Verification items for the finished model (mm, model axes). A direction names the side the tool comes from. Coordinates: 2 decimals unless noted, no trailing zeros. Loops run counter-clockwise (first coordinate to the right, second up) from the corner with the lowest first, then second, coordinate; pieces in that order, holes last. Notation, with made-up numbers: (51.5, 15) - (86.5, 15) arc R19 cw to (86.5, 36) - close; hole circle Ø7 at (-21, 44). An arc over 180 degrees is marked (long way). One line per item, written item: value. Start each with the question number.
(1) Draft check along X on faces 4 (the face through (177.8, 2, 49)), 5 (the face through (144.14, -2.11, 42.1)). Enter one of: +X half, -X half, draft (parallel to the pull), parting line (faces both ways), or undercut.
(2) Set-up check for faces 1 (the face through (63.5, 2, 2)), 2 (the face through (44, 2, 47.625)), 3 (the face through (159, 2, 50.8)): record each of +Z, -Z, +X, -X, +Y, -Y from which the full face is reachable in a straight line by a thin tool's end or side.
(3) Section check B-B (x = 106). Record the boundary of the cut face in (y, z) (3 decimals), plus the area to 3 significant figures.
(4) Section check C-C (x = 173.5). Record the boundary of the cut face in (y, z) (3 decimals), plus the area to 3 significant figures.
(5) Section check D-D (x = 27.5). Record the boundary of the cut face in (y, z) (3 decimals), plus the area to 3 significant figures.
(6) Thickness scan on probe 1 along X at (y, z) = (2.9, 24); probe 2 along Y at (x, z) = (130, 36.5) (3 decimals); probe 3 along X at (y, z) = (0.5, 42.5). Record the ranges inside material, lowest first. Write a range as [from, to].
(7) Gauge pin test, flat ends, axial feed: P1, Ø1.5, axis at y = 1.5, z = 27, coming from the -X side; P2, Ø1, axis at x = 146.5, y = 1, coming from the -Z side (3 decimals); P3, Ø0.8, axis at y = -1, z = 34.5, coming from the +X side. Record the tip position at first contact, or that the pin passes through.
(8) Section check A-A (z = 14.5). Record the boundary of the cut face in (x, y) (3 decimals).
```python
from build123d import *

# Parameters (mm, degrees)
BOSS_EXTRUDE1_DEPTH = 3.175
SKETCH2_W           = 12.7
SKETCH2_H           = 6.35
CUT_EXTRUDE1_DEPTH  = 198.182581951
SKETCH3_W           = 19.05
SKETCH3_H           = 3.175
BOSS_EXTRUDE2_DEPTH = 6.35
CUT_EXTRUDE4_DEPTH  = 3.175
SKETCH6_W           = 3.74
SKETCH6_H           = 38.1
BOSS_EXTRUDE3_DEPTH = 2.54
FILLET1_R           = 5.08
CUT_EXTRUDE5_REACH  = 113.371
SKETCH7_W           = 29.301181898
SKETCH7_H           = 1.2
FILLET3_R           = 2.54


with BuildPart() as part:
    # Sketch1 → Boss-Extrude1 (new body)
    with BuildSketch(Plane(origin=(0, 0, 0), x_dir=(1, 0, 0), z_dir=(0, 1, 0))):
        Polygon((12.7, 0), (0, 0), (0, -50.8), (12.7, -50.8), (12.7, -47.625), (25.4, -47.625), (25.4, -50.8), (38.1, -50.8), (38.1, -47.625), (50.8, -47.625), (50.8, -50.8), (63.5, -50.8), (63.5, -47.625), (76.2, -47.625), (76.2, -50.8), (88.9, -50.8), (88.9, -47.625), (101.6, -47.625), (101.6, -50.8), (114.3, -50.8), (114.3, -47.625), (127, -47.625), (127, -50.8), (139.7, -50.8), (139.7, -47.625), (152.4, -47.625), (152.4, -50.8), (165.1, -50.8), (165.1, -47.625), (177.8, -47.625), (177.8, -50.8), (190.5, -50.8), (190.5, 0), (177.8, 0), (177.8, -3.175), (165.1, -3.175), (165.1, 0), (152.4, 0), (152.4, -3.175), (139.7, -3.175), (139.7, 0), (127, 0), (127, -3.175), (114.3, -3.175), (114.3, 0), (101.6, 0), (101.6, -3.175), (88.9, -3.175), (88.9, 0), (76.2, 0), (76.2, -3.175), (63.5, -3.175), (63.5, 0), (50.8, 0), (50.8, -3.175), (38.1, -3.175), (38.1, 0), (25.4, 0), (25.4, -3.175), (12.7, -3.175), align=None)
    extrude(amount=BOSS_EXTRUDE1_DEPTH)

    # Sketch2 → Cut-Extrude1 (cut, through all)
    with BuildSketch(Plane(origin=(0, 3.175, 0), x_dir=(1, 0, 0), z_dir=(0, 1, 0))):
        with Locations((6.35, -25.4)):
            Rectangle(SKETCH2_W, SKETCH2_H)
    extrude(amount=-CUT_EXTRUDE1_DEPTH, mode=Mode.SUBTRACT)

    # Sketch3 → Boss-Extrude2 (add)
    with BuildSketch(Plane.ZY):
        with Locations((12.7, 1.5875)):
            Rectangle(SKETCH3_W, SKETCH3_H)
        with Locations((38.1, 1.5875)):
            Rectangle(SKETCH3_W, SKETCH3_H)
    extrude(amount=BOSS_EXTRUDE2_DEPTH)

    # Sketch5 → Cut-Extrude4 (cut)
    with BuildSketch(Plane(origin=(0, 3.175, 0), x_dir=(1, 0, 0), z_dir=(0, 1, 0))):
        with BuildLine():
            Line((82.48, -6.35), (82.48, -44.45))
            ThreePointArc((82.48, -44.45), (81.28, -45.65), (80.08, -44.45))
            Line((80.08, -44.45), (80.08, -6.35))
            ThreePointArc((80.08, -6.35), (81.28, -5.15), (82.48, -6.35))
        make_face()
    extrude(amount=-CUT_EXTRUDE4_DEPTH, mode=Mode.SUBTRACT)

    # Sketch6 → Boss-Extrude3 (add)
    with BuildSketch(Plane(origin=(0, 0, 0), x_dir=(-1, 0, 0), z_dir=(0, -1, 0))):
        with Locations((-106.01, -25.4)):
            Rectangle(SKETCH6_W, SKETCH6_H)
        with Locations((-93.31, -25.4)):
            Rectangle(SKETCH6_W, SKETCH6_H)
        with Locations((-118.71, -25.4)):
            Rectangle(SKETCH6_W, SKETCH6_H)
        with Locations((-131.41, -25.4)):
            Rectangle(SKETCH6_W, SKETCH6_H)
        with Locations((-144.11, -25.4)):
            Rectangle(SKETCH6_W, SKETCH6_H)
    extrude(amount=BOSS_EXTRUDE3_DEPTH)

    # Fillet1
    # the kernel refuses this fillet: 5.08 mm, written as the material it takes off along each edge
    with BuildSketch(Plane(origin=(106.178522628, -2.54, 6.35), x_dir=(0, 1, 0), z_dir=(-1, 0, 0)), Plane(origin=(80.441477372, -2.54, 44.45), x_dir=(0, 1, 0), z_dir=(1, 0, 0))) as fillet1_piece_1:
        with BuildLine():
            CenterArc((5.08, -4.399409051), FILLET1_R, 120, 60)
            Line((0, -4.399409051), (-0.1016, -4.399409051))
            Line((-0.1016, -4.399409051), (-0.1016, 0))
            Line((-0.1016, 0), (0, 0.1016))
            ThreePointArc((0, 0.1016), (1.27, 0.1016), (2.4892, 0.087988181))
            Line((2.4892, 0.087988181), (2.54, 0))
        make_face()
    extrude(amount=25.737045256, mode=Mode.SUBTRACT)
    with BuildSketch(Plane(origin=(93.141477372, -2.54, 6.35), x_dir=(0, 1, 0), z_dir=(1, 0, 0)), Plane(origin=(105.841477372, -2.54, 6.35), x_dir=(0, 1, 0), z_dir=(1, 0, 0)), Plane(origin=(118.541477372, -2.54, 6.35), x_dir=(0, 1, 0), z_dir=(1, 0, 0)), Plane(origin=(131.241477372, -2.54, 6.35), x_dir=(0, 1, 0), z_dir=(1, 0, 0)), Plane(origin=(156.978522628, -2.54, 44.45), x_dir=(0, 1, 0), z_dir=(-1, 0, 0)), Plane(origin=(144.278522628, -2.54, 44.45), x_dir=(0, 1, 0), z_dir=(-1, 0, 0)), Plane(origin=(131.578522628, -2.54, 44.45), x_dir=(0, 1, 0), z_dir=(-1, 0, 0)), Plane(origin=(118.878522628, -2.54, 44.45), x_dir=(0, 1, 0), z_dir=(-1, 0, 0))) as fillet1_piece_2:
        with BuildLine():
            CenterArc((5.08, 4.399409051), FILLET1_R, 180, 60)
            Line((0, 4.399409051), (-0.1016, 4.399409051))
            Line((-0.1016, 4.399409051), (-0.1016, 0))
            Line((-0.1016, 0), (0, -0.1016))
            ThreePointArc((0, -0.1016), (1.27, -0.1016), (2.4892, -0.087988181))
            Line((2.4892, -0.087988181), (2.54, 0))
        make_face()
    extrude(amount=25.737045256, mode=Mode.SUBTRACT)

    # Cut-Extrude5: up to this face of the body (flat: up to its plane)
    cut_extrude5_end = Plane(part.part.faces().sort_by_distance((145.98, -1.229881831, 25.4))[0])
    # Sketch7 → Cut-Extrude5 (cut, up to the picked face)
    with BuildSketch(Plane.ZY.offset(-91.44), mode=Mode.PRIVATE) as cut_extrude5_sk1:
        with Locations((25.4, -0.6)):
            Rectangle(SKETCH7_W, SKETCH7_H)
    cut_extrude5_tool1 = split(extrude(cut_extrude5_sk1.sketch, amount=-CUT_EXTRUDE5_REACH, mode=Mode.PRIVATE), bisect_by=cut_extrude5_end, keep=Keep.BOTH, mode=Mode.PRIVATE)
    add(cut_extrude5_tool1.solids().sort_by(Axis((91.44, -0.6, 25.4), (1, 0, 0)))[0], mode=Mode.SUBTRACT)

    # Fillet3
    # the kernel refuses this fillet: 2.54 mm, written as the material it adds along each edge
    with BuildSketch(Plane(origin=(120.58, 0, 6.35), x_dir=(0, 0, -1), z_dir=(-1, 0, 0)), Plane(origin=(116.84, 0, 44.45), x_dir=(0, 0, 1), z_dir=(1, 0, 0)), Plane(origin=(107.88, 0, 6.35), x_dir=(0, 0, -1), z_dir=(-1, 0, 0)), Plane(origin=(104.14, 0, 44.45), x_dir=(0, 0, 1), z_dir=(1, 0, 0)), Plane(origin=(95.18, 0, 6.35), x_dir=(0, 0, -1), z_dir=(-1, 0, 0)), Plane(origin=(91.44, 0, 44.45), x_dir=(0, 0, 1), z_dir=(1, 0, 0)), Plane(origin=(145.98, 0, 6.35), x_dir=(0, 0, -1), z_dir=(-1, 0, 0)), Plane(origin=(142.24, 0, 44.45), x_dir=(0, 0, 1), z_dir=(1, 0, 0)), Plane(origin=(133.28, 0, 6.35), x_dir=(0, 0, -1), z_dir=(-1, 0, 0)), Plane(origin=(129.54, 0, 44.45), x_dir=(0, 0, 1), z_dir=(1, 0, 0))) as fillet3_piece_1:
        with BuildLine():
            CenterArc((1.280203612, 2.54), FILLET3_R, 221.810314896, 48.189685104)
            ThreePointArc((-0.613000609, 0.846666667), (-0.284665667, 0.439141971), (0, 0))
            Line((0, 0), (1.280203612, 0))
        make_face()
    extrude(amount=3.74)


solid = part.part
```
Responses:
1. face 4: undercut
1. face 5: draft
2. face 1: -Z, +Y, -Y
2. face 2: +Z, +Y, -Y
2. face 3: +Z, +X, -X, +Y, -Y
3. outline: (-2.54, 10.749) arc R5.08 ccw to (-0.847, 6.963) arc R2.54 cw to (0, 5.07) - (0, 0) - (3.175, 0) - (3.175, 50.8) - (0, 50.8) - (0, 45.73) arc R2.54 cw to (-0.847, 43.837) arc R5.08 ccw to (-2.54, 40.051) - close; hole (-1.2, 10.749) - (0, 10.749) - (0, 40.051) - (-1.2, 40.051) - close
3. area: 217 mm²
4. outline: (0, 3.175) - (3.175, 3.175) - (3.175, 47.625) - (0, 47.625) - close
4. area: 141 mm²
5. outline: (0, 0) - (3.175, 0) - (3.175, 50.8) - (0, 50.8) - close
5. area: 161 mm²
6. probe 1: x = [12.7, 80.08], [82.48, 190.5]
6. probe 2: y = [-2.54, -1.2], [0, 3.175]
6. probe 3: x = [-6.35, 80.08], [82.48, 190.5]
7. P1: stops at x = 12.7
7. P2: stops at z = 3.175
7. P3: stops at x = 145.98
8. outline: (-6.35, 0) - (80.08, 0) - (80.08, 3.175) - (-6.35, 3.175) - close; (82.48, 0) - (190.5, 0) - (190.5, 3.175) - (82.48, 3.175) - close; (91.44, -2.54) - (95.18, -2.54) - (95.18, -1.2) - (91.44, -1.2) - close; (104.14, -2.54) - (107.88, -2.54) - (107.88, -1.2) - (104.14, -1.2) - close; (116.84, -2.54) - (120.58, -2.54) - (120.58, -1.2) - (116.84, -1.2) - close; (129.54, -2.54) - (133.28, -2.54) - (133.28, -1.2) - (129.54, -1.2) - close; (142.24, -2.54) - (145.98, -2.54) - (145.98, -1.2) - (142.24, -1.2) - close
